Here's how the part is built. I have some questions about the finished solid (model axes, mm). A direction names the side the tool comes from. Give positions to 0.01 mm unless a question says otherwise; leave off trailing zeros. Loops run counter-clockwise (first coordinate to the right, second up) from the corner with the lowest first, then second, coordinate; pieces in that order, holes last.
Q1. If we section it at C-C (y = 9): Please give me the cut outline in (x, z).
Q2. If we section it at D-D (x = -8.5): Please give me the cut outline in (y, z), plus the area to 3 significant figures.
Q3. We'd pull the mould along Y, two halves only. Please class faces 1 (the face through (-8.6, 5.58, -5.27)), 2 (the face through (-5, 3, 8.517)), 3 (the face through (-2, 0, 1)): +Y half, -Y half, draft (parallel to the pull), parting line (faces both ways), or undercut.
Q4. I need wall thicknesses on line 1 (Z direction, x = -6.5, y = 5); line 2 (Y direction, x = -2.5, z = 7.5); line 3 (X direction, y = 4.75, z = -4.5). Which ranges of each line are inside material? Lowest first, please.
Q5. If we section it at A-A (z = 7.75): Please give me the cut outline in (x, y), plus the area to 3 significant figures.
Q6. Will these pins go through, and if not, where does the flat tip stop? P1, Ø1.5, axis at x = -5.5, z = -1, coming from the +Y side; P2, Ø1.5, axis at x = 2, z = 4.5, coming from the -Y side; P3, Ø2.5, axis at y = 6, z = 7, coming from the +X side.
Q7. If we section it at B-B (y = 6): Please give me the cut outline in (x, z).
Q8. For faces 4 (the face through (-6.334, 5, -5)), 5 (the face through (-12.334, 3, 1)), 6 (the face through (-8, 5.7, -4.083)), which set-ups out of +Z, -Z, +X, -X, +Y, -Y let a thin tool reach every point of the face, with its end or its side?
from build123d import *

# Parameters (mm, degrees)
SKETCH_1_W          = 20
SKETCH_1_H          = 15
EXTRUDE_2_DEPTH     = 4
SKETCH_3_W          = 6
SKETCH_3_H          = 15
EXTRUDE_3_DEPTH     = 6
SKETCH_4_W          = 6
SKETCH_4_H          = 10.2
CUT_EXTRUDE_1_DEPTH = 6
SKETCH_5_R          = 1.6
CUT_EXTRUDE_2_DEPTH = 21


with BuildPart() as part:
    # 草图1 → 凸台-拉伸2 (new body)
    with BuildSketch(Plane(origin=(0, 0, 0), x_dir=(1, 0, 0), z_dir=(0, 1, 0))):
        with Locations((-2.334337349, -1.016566265)):
            Rectangle(SKETCH_1_W, SKETCH_1_H)
    extrude(amount=EXTRUDE_2_DEPTH)

    # 草图3 → 凸台-拉伸3 (add)
    with BuildSketch(Plane(origin=(0, 4, 0), x_dir=(1, 0, 0), z_dir=(0, 1, 0))):
        with Locations((-9.334337349, -1.016566265)):
            Rectangle(SKETCH_3_W, SKETCH_3_H)
    extrude(amount=EXTRUDE_3_DEPTH)

    # 草图4 → 切除-拉伸1 (cut)
    with BuildSketch(Plane(origin=(0, 10, 0), x_dir=(1, 0, 0), z_dir=(0, 1, 0))):
        with Locations((-9.334337349, -1.016566265)):
            Rectangle(SKETCH_4_W, SKETCH_4_H)
    extrude(amount=-CUT_EXTRUDE_1_DEPTH, mode=Mode.SUBTRACT)

    # 草图5 → 切除-拉伸2 (cut)
    with BuildSketch(Plane.XY.offset(8.516566265)):
        with Locations((-9.334337349, 7)):
            Circle(SKETCH_5_R)
        with BuildLine():
            Line((-9.334337349, 10), (-12.334337349, 10))
            Line((-12.334337349, 10), (-12.334337349, 7))
            ThreePointArc((-12.334337349, 7), (-11.455657693, 9.121320344), (-9.334337349, 10))
        make_face()
        with BuildLine():
            Line((-6.334337349, 10), (-9.334337349, 10))
            ThreePointArc((-9.334337349, 10), (-7.213017006, 9.121320344), (-6.334337349, 7))
            Line((-6.334337349, 7), (-6.334337349, 10))
        make_face()
    extrude(amount=-CUT_EXTRUDE_2_DEPTH, mode=Mode.SUBTRACT)


solid = part.part
Check sheet entries:
1. outline: (-11.57, -6.48) - (-7.1, -6.48) - (-7.1, -4.08) - (-11.57, -4.08) - close; (-11.57, 6.12) - (-7.1, 6.12) - (-7.1, 8.52) - (-11.57, 8.52) - close
2. outline: (0, -6.48) - (5.63, -6.48) - (5.63, -4.08) - (4, -4.08) - (4, 6.12) - (5.63, 6.12) - (5.63, 8.52) - (0, 8.52) - close; (8.37, -6.48) - (9.88, -6.48) - (9.88, -4.08) - (8.37, -4.08) - close; (8.37, 6.12) - (9.88, 6.12) - (9.88, 8.52) - (8.37, 8.52) - close
2. area: 75.1 mm2
3. face 1: undercut
3. face 2: draft
3. face 3: -Y half
4. line 1: z = -6.48 to -4.08, 6.12 to 8.52
4. line 2: y = 0 to 4
4. line 3: x = -12.33 to -6.33
5. outline: (-12.33, 0) - (7.67, 0) - (7.67, 4) - (-6.33, 4) - (-6.33, 7) arc R3 ccw to (-12.33, 7) - close; hole circle Ø3.2 at (-9.33, 7)
5. area: 104 mm2
6. P1: stops at y = 4
6. P2: stops at y = 0
6. P3: stops at x = -6.33
7. outline: (-12.33, -6.48) - (-10.58, -6.48) - (-10.58, -4.08) - (-12.33, -4.08) - close; (-12.33, 6.12) - (-10.58, 6.12) - (-10.58, 8.52) - (-12.33, 8.52) - close; (-8.09, -6.48) - (-6.33, -6.48) - (-6.33, -4.08) - (-8.09, -4.08) - close; (-8.09, 6.12) - (-6.33, 6.12) - (-6.33, 8.52) - (-8.09, 8.52) - close
8. face 4: +Z, -Z, +X, +Y
8. face 5: +Z, -Z, -X, +Y, -Y
8. face 6: +X, -X, +Y
